```python
from build123d import *

# Parameters (mm, degrees)
BOSS_EXTRUDE1_DEPTH = 3.175
SKETCH3_R           = 1.5
CUT_EXTRUDE1_DEPTH  = 3.175


with BuildPart() as part:
    # Sketch1 → Boss-Extrude1 (new body)
    with BuildSketch(Plane.XY):
        Polygon((-114.3, 127), (-114.3, 114.3), (-111.125, 114.3), (-111.125, 101.6), (-114.3, 101.6), (-114.3, 88.9), (-111.125, 88.9), (-111.125, 76.2), (-114.3, 76.2), (-114.3, 63.5), (-111.125, 63.5), (-111.125, 50.8), (-114.3, 50.8), (-114.3, 38.1), (-111.125, 38.1), (-111.125, 25.4), (-114.3, 25.4), (-114.3, 12.7), (-111.125, 12.7), (-111.125, 0), (-114.3, 0), (-114.3, -12.7), (-111.125, -12.7), (-111.125, -25.4), (-114.3, -25.4), (-114.3, -38.1), (-111.125, -38.1), (-111.125, -50.8), (-114.3, -50.8), (-114.3, -63.5), (-111.125, -63.5), (-111.125, -76.2), (-114.3, -76.2), (-114.3, -88.9), (-111.125, -88.9), (-111.125, -101.6), (-114.3, -101.6), (-114.3, -114.3), (-111.125, -114.3), (-111.125, -127), (-95.25, -127), (-95.25, -133.35), (-57.15, -133.35), (-57.15, -127), (-19.05, -127), (-19.05, -133.35), (19.05, -133.35), (19.05, -127), (57.15, -127), (57.15, -133.35), (95.25, -133.35), (95.25, -127), (111.125, -127), (111.125, -114.3), (114.3, -114.3), (114.3, -101.6), (111.125, -101.6), (111.125, -88.9), (114.3, -88.9), (114.3, -76.2), (111.125, -76.2), (111.125, -63.5), (114.3, -63.5), (114.3, -50.8), (111.125, -50.8), (111.125, -38.1), (114.3, -38.1), (114.3, -25.4), (111.125, -25.4), (111.125, -12.7), (114.3, -12.7), (114.3, 0), (111.125, 0), (111.125, 12.7), (114.3, 12.7), (114.3, 25.4), (111.125, 25.4), (111.125, 38.1), (114.3, 38.1), (114.3, 50.8), (111.125, 50.8), (111.125, 63.5), (114.3, 63.5), (114.3, 76.2), (111.125, 76.2), (111.125, 88.9), (114.3, 88.9), (114.3, 101.6), (111.125, 101.6), (111.125, 114.3), (114.3, 114.3), (114.3, 127), align=None)
    extrude(amount=BOSS_EXTRUDE1_DEPTH)

    # Sketch3 → Cut-Extrude1 (cut)
    with BuildSketch(Plane(origin=(0, 0, 0), x_dir=(-1, 0, 0), z_dir=(0, 0, -1))):
        with Locations((-95.25, 112)):
            Circle(SKETCH3_R)
        with Locations((-95.25, 96.25)):
            Circle(SKETCH3_R)
        with Locations((95.25, 96.25)):
            Circle(SKETCH3_R)
        with Locations((95.25, 112)):
            Circle(SKETCH3_R)
    extrude(amount=-CUT_EXTRUDE1_DEPTH, mode=Mode.SUBTRACT)


solid = part.part
```
Model file for the job. Use its own axes, mm. Give positions to 0.01 mm unless a question says otherwise; leave off trailing zeros. Order: outer loops, then holes, each group sorted by start corner. A loop starts at its lowest first (then second) coordinate and runs counter-clockwise, first axis right, second up.
1) Wall check: probe 1 along X at (y, z) = (112, 1.35) (3 decimals); probe 2 along X at (y, z) = (96.25, 2.1); probe 3 along X at (y, z) = (-23.5, 1.3) (3 decimals). Give the ranges that are in metal, low to high.
2) Saw through at B-B, the plane z = 0.8. Count the separate pieces of the cut face and the enclosed holes in it, then the cut area to 3 significant figures.
3) Saw through at A-A, the plane y = 84.5. Write the cut outline in (x, z) (3 decimals), then the cut area to 3 significant figures.
4) Pin check, flat tips, straight feed: pin 1 (1.6 mm diameter, centred on y = -131, z = 1, fed in from -X); pin 2 (1 mm diameter, centred on y = 105.5, z = 2, fed in from +X) (3 decimals); pin 3 (1 mm diameter, centred on x = -35, z = 2, fed in from -Y). Stop position of each tip, or through.
Computed:
1. probe 1: x = -111.125 to -96.75, -93.75 to 93.75, 96.75 to 111.125
1. probe 2: x = -114.3 to -96.75, -93.75 to 93.75, 96.75 to 114.3
1. probe 3: x = -111.125 to 111.125
2. separate pieces: 1
2. enclosed holes: 4
2. area: 58,000 mm2
3. outline: (-111.125, 0) - (111.125, 0) - (111.125, 3.175) - (-111.125, 3.175) - close
3. area: 706 mm2
4. pin 1: stops at x = -95.25
4. pin 2: stops at x = 111.125
4. pin 3: stops at y = -127
